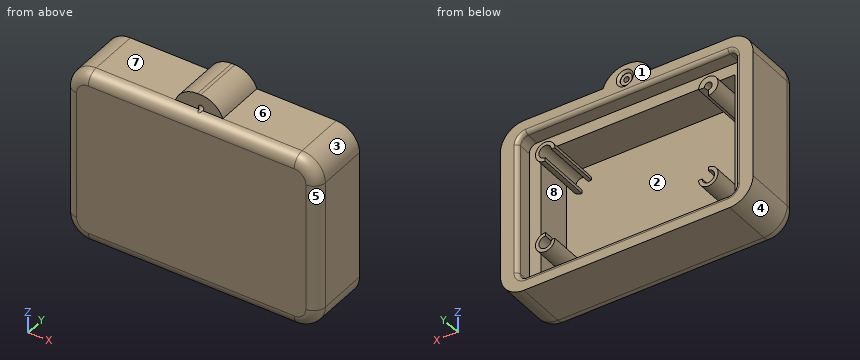
from build123d import *

# Parameters (mm, degrees)
SKETCH1_W               = 82.55
SKETCH1_H               = 57.15
BOSS_EXTRUDE1_DEPTH     = 20.32
FILLET2_R               = 7.62
FILLET3_R               = 3.81
SKETCH2_W               = 63.5
SKETCH2_H               = 40.64
CUT_EXTRUDE1_DEPTH      = 17.78
SKETCH9_W               = 15.46152766
SKETCH9_H               = 16.51
BOSS_EXTRUDE5_DEPTH     = 5.08
FILLET10_R              = 7.62
SKETCH7_W               = 71.12
SKETCH7_H               = 48.26
CUT_EXTRUDE4_DEPTH      = 5.461
FILLET12_R              = 2.54
FILLET13_R              = 1.27
SKETCH5_R               = 3.175
BOSS_EXTRUDE6_DEPTH     = 17.78
SKETCH11_R              = 1.27
SKETCH11_R_2            = 2.032
CUT_EXTRUDE5_DEPTH      = 17.78
CUT_EXTRUDE_THIN1_DEPTH = 102.964471319


with BuildPart() as part:
    # Sketch1 → Boss-Extrude1 (new body)
    with BuildSketch(Plane(origin=(0, 0, 0), x_dir=(1, 0, 0), z_dir=(0, 1, 0))):
        with Locations((41.275, 28.575)):
            Rectangle(SKETCH1_W, SKETCH1_H)
    extrude(amount=BOSS_EXTRUDE1_DEPTH)

    # Fillet2
    fillet2_edges = [part.edges().sort_by_distance(p)[0] for p in [
        (0, 10.16, -57.15),
        (82.55, 10.16, -57.15),
        (82.55, 10.16, 0),
        (0, 10.16, 0),
    ]]
    fillet(fillet2_edges, radius=FILLET2_R)

    # Fillet3
    fillet3_edges = [part.edges().sort_by_distance(p)[0] for p in [
        (41.275, 0, -57.15),
        (0, 0, -28.575),
        (82.55, 0, -28.575),
        (41.275, 0, 0),
        (2.231846327, 0, -54.918153673),
        (2.231846327, 0, -2.231846327),
        (80.318153673, 0, -2.231846327),
        (80.318153673, 0, -54.918153673),
    ]]
    fillet(fillet3_edges, radius=FILLET3_R)

    # Sketch2 → Cut-Extrude1 (cut)
    with BuildSketch(Plane(origin=(0, 20.32, 0), x_dir=(1, 0, 0), z_dir=(0, 1, 0))):
        with Locations((41.275, 28.575)):
            Rectangle(SKETCH2_W, SKETCH2_H)
    extrude(amount=-CUT_EXTRUDE1_DEPTH, mode=Mode.SUBTRACT)

    # Sketch9 → Boss-Extrude5 (add)
    with BuildSketch(Plane.XY):
        with Locations((41.275, 12.065)):
            Rectangle(SKETCH9_W, SKETCH9_H)
    extrude(amount=BOSS_EXTRUDE5_DEPTH)

    # Fillet10
    # the kernel refuses this fillet: 7.62 mm, written as the material it takes off along each edge
    with BuildSketch(Plane(origin=(49.00576383, -14.150512242, 5.08), x_dir=(-1, 0, 0), z_dir=(0, 1, 0))) as fillet10_piece_1:
        with BuildLine():
            CenterArc((7.184204897, -7.62), FILLET10_R, 90, 70.528779366)
            Line((0, -5.08), (-0.143684098, -5.0292))
            ThreePointArc((-0.143684098, -5.0292), (-0.1524, -2.54), (-0.1524, 0))
            Line((-0.1524, 0), (0, 0.1524))
            Line((0, 0.1524), (7.184204897, 0.1524))
            Line((7.184204897, 0.1524), (7.184204897, 0))
        make_face()
    extrude(amount=52.431024484, mode=Mode.SUBTRACT)
    with BuildSketch(Plane(origin=(33.54423617, 38.280512242, 5.08), x_dir=(0, 0, -1), z_dir=(0, -1, 0))) as fillet10_piece_2:
        with BuildLine():
            CenterArc((7.62, 7.184204897), FILLET10_R, 180, 70.528779366)
            Line((0, 7.184204897), (-0.1524, 7.184204897))
            Line((-0.1524, 7.184204897), (-0.1524, 0))
            Line((-0.1524, 0), (0, -0.1524))
            ThreePointArc((0, -0.1524), (2.54, -0.1524), (5.0292, -0.143684098))
            Line((5.0292, -0.143684098), (5.08, 0))
        make_face()
    extrude(amount=52.431024484, mode=Mode.SUBTRACT)

    # Sketch7 → Cut-Extrude4 (cut)
    with BuildSketch(Plane(origin=(0, 20.32, 0), x_dir=(1, 0, 0), z_dir=(0, 1, 0))):
        with Locations((41.275, 28.575)):
            Rectangle(SKETCH7_W, SKETCH7_H)
    extrude(amount=-CUT_EXTRUDE4_DEPTH, mode=Mode.SUBTRACT)

    # Fillet12
    fillet12_edges = [part.edges().sort_by_distance(p)[0] for p in [
        (5.715, 17.5895, -52.705),
        (76.835, 17.5895, -52.705),
        (76.835, 17.5895, -4.445),
        (5.715, 17.5895, -4.445),
    ]]
    fillet(fillet12_edges, radius=FILLET12_R)

    # Fillet13
    fillet13_edges = [part.edges().sort_by_distance(p)[0] for p in [
        (41.275, 20.32, -52.705),
        (76.835, 20.32, -28.575),
        (41.275, 20.32, -4.445),
        (5.715, 20.32, -28.575),
        (76.091051224, 20.32, -51.961051224),
        (76.091051224, 20.32, -5.188948776),
        (6.458948776, 20.32, -51.961051224),
        (6.458948776, 20.32, -5.188948776),
    ]]
    fillet(fillet13_edges, radius=FILLET13_R)

    # Sketch5 → Boss-Extrude6 (add)
    with BuildSketch(Plane(origin=(0, 2.54, 0), x_dir=(1, 0, 0), z_dir=(0, 1, 0))):
        with Locations(Location((14.605, 43.815, 0), (0, 0, 90))):
            Circle(SKETCH5_R)
        with Locations(Location((14.605, 13.335, 0), (0, 0, 90))):
            Circle(SKETCH5_R)
        with Locations(Location((67.945, 43.815, 0), (0, 0, 90))):
            Circle(SKETCH5_R)
        with Locations(Location((67.945, 13.335, 0), (0, 0, 90))):
            Circle(SKETCH5_R)
    extrude(amount=BOSS_EXTRUDE6_DEPTH)

    # Sketch11 → Cut-Extrude5 (cut)
    with BuildSketch(Plane(origin=(0, 20.32, 0), x_dir=(1, 0, 0), z_dir=(0, 1, 0))):
        with Locations(Location((14.605, 13.335, 0), (0, 0, 270))):
            Circle(SKETCH11_R)
        with Locations(Location((14.605, 43.815, 0), (0, 0, 270))):
            Circle(SKETCH11_R_2)
        with Locations(Location((67.945, 13.335, 0), (0, 0, 270))):
            Circle(SKETCH11_R_2)
        with Locations(Location((67.945, 43.815, 0), (0, 0, 270))):
            Circle(SKETCH11_R_2)
    extrude(amount=-CUT_EXTRUDE5_DEPTH, mode=Mode.SUBTRACT)

    # Sketch17 → Cut-Extrude-Thin1 (cut, through all)
    with BuildSketch(Plane(origin=(0, 2.54, 0), x_dir=(1, 0, 0), z_dir=(0, 1, 0))):
        with BuildLine():
            ThreePointArc((67.801605081, 40.643239779), (65.547471879, 41.576932323), (64.613779335, 43.831065525))
            Line((64.613779335, 43.831065525), (67.153779335, 43.831065525))
            ThreePointArc((67.153779335, 43.831065525), (67.343523103, 43.372983547), (67.801605081, 43.183239779))
            Line((67.801605081, 43.183239779), (67.801605081, 40.643239779))
        make_face()
        with BuildLine():
            ThreePointArc((64.77, 13.335), (65.69993597, 15.58006403), (67.945, 16.51))
            Line((67.945, 16.51), (67.945, 13.97))
            ThreePointArc((67.945, 13.97), (67.495987194, 13.784012806), (67.31, 13.335))
            Line((67.31, 13.335), (64.77, 13.335))
        make_face()
        with BuildLine():
            ThreePointArc((17.78, 43.815), (16.85006403, 41.56993597), (14.605, 40.64))
            Line((14.605, 40.64), (14.605, 43.18))
            ThreePointArc((14.605, 43.18), (15.054012806, 43.365987194), (15.24, 43.815))
            Line((15.24, 43.815), (17.78, 43.815))
        make_face()
        with BuildLine():
            ThreePointArc((14.605, 16.51), (16.85006403, 15.58006403), (17.78, 13.335))
            Line((17.78, 13.335), (15.24, 13.335))
            ThreePointArc((15.24, 13.335), (15.054012806, 13.784012806), (14.605, 13.97))
            Line((14.605, 13.97), (14.605, 16.51))
        make_face()
    extrude(amount=CUT_EXTRUDE_THIN1_DEPTH, mode=Mode.SUBTRACT)

    # Sketch19 → CBORE for #0 Binding Head Machine Screw1 (revolve, cut)
    with BuildSketch(Plane(origin=(41.911122971, 20.32, 0.674781491), x_dir=(0, 0, 1), z_dir=(1, 0, 0))):
        Polygon((0, 0), (0, 20.32), (0.889, 20.32), (0.889, 0.8128), (1.98501, 0.8128), (1.98501, 0.668166645), (2.7813, 0), align=None)
    revolve(axis=Axis((41.911122971, 26.67, 0.674781491), (0, -1, 0)), mode=Mode.SUBTRACT)


solid = part.part
Could you check a few things on this model? Use its own coordinates, in mm. Face numbers are marked on the shaded views. A direction names the side the tool comes from. Coordinates: 2 decimals unless noted, no trailing zeros. Order: outer loops, then holes, each group sorted by start corner. A loop starts at its lowest first (then second) coordinate and runs counter-clockwise, first axis right, second up.
Q1. Which directions (+Z, -Z, +X, -X, +Y, -Y) give clear straight access to the entire face, cutting with the end or side of a thin tool? Please do the marked faces 5, 6, 7 and 8.
Q2. Suppose I cut it at C-C on z = -28. Please give me the cut outline in (x, y) (3 decimals).
Q3. Suppose I cut it at B-B on x = 21. Please give me the cut outline in (y, z) (3 decimals).
Q4. Suppose I cut it at A-A on y = 5.5. Give the number of separate pieces and of enclosed holes in the cut face, and give its area (3 significant figures).
Q5. Will these pins go through, and if not, where does the flat tip stop? pin 1 (4 mm diameter, centred on x = 43.5, z = -27.5, fed in from +Y); pin 2 (10 mm diameter, centred on x = 73, z = -23, fed in from +Y); pin 3 (3 mm diameter, centred on x = 41.91, z = 0.67, fed in from -Y).
Q6. Thinking about a two-plate mould opening in X: for the marked faces 1, 2, 3 and 4, which applies, released by +X, released by -X, zero draft, split by the parting line, or undercut?
Q7. Please list where these lines run through material, in increasing order: L1, parallel to Z at x = 32, y = 11.5 (3 decimals); L2, parallel to Z at x = 57, y = 16.5 (3 decimals); L3, parallel to X at y = 14, z = -44 (3 decimals).
Answer:
1. face 5: +Z, -Z, +X, -Y
1. face 6: +Z, +X, +Y, -Y
1. face 7: +Z, -X, +Y, -Y
1. face 8: +Y
2. outline: (0, 3.81) arc R3.81 ccw to (3.81, 0) - (78.74, 0) arc R3.81 ccw to (82.55, 3.81) - (82.55, 20.32) - (78.105, 20.32) arc R1.27 ccw to (76.835, 19.05) - (76.835, 14.859) - (73.025, 14.859) - (73.025, 2.54) - (9.525, 2.54) - (9.525, 14.859) - (5.715, 14.859) - (5.715, 19.05) arc R1.27 ccw to (4.445, 20.32) - (0, 20.32) - close
3. outline: (0, -53.34) arc R3.81 ccw to (3.81, -57.15) - (20.32, -57.15) - (20.32, -53.975) arc R1.27 ccw to (19.05, -52.705) - (14.859, -52.705) - (14.859, -48.895) - (2.54, -48.895) - (2.54, -8.255) - (14.859, -8.255) - (14.859, -4.445) - (19.05, -4.445) arc R1.27 ccw to (20.32, -3.175) - (20.32, 0) - (3.81, 0) arc R3.81 ccw to (0, -3.81) - close
4. separate pieces: 5
4. enclosed holes: 2
4. area: 2,210 mm2
5. pin 1: stops at y = 2.54
5. pin 2: stops at y = 20.32
5. pin 3: stops at y = 1.44
6. face 1: zero draft
6. face 2: undercut
6. face 3: released by +X
6. face 4: released by -X
7. L1: z = -57.15 to -48.895, -8.255 to 0
7. L2: z = -57.15 to -52.705, -4.445 to 0
7. L3: x = 0 to 9.525, 11.435 to 12.581, 16.629 to 17.775, 64.775 to 65.921, 69.969 to 71.115, 73.025 to 82.55
